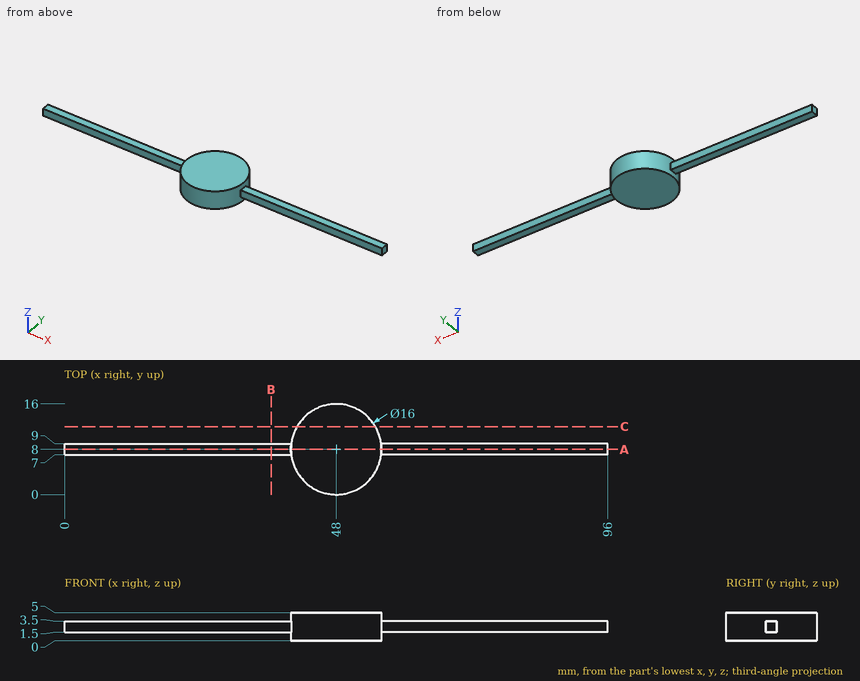
Input: dimensioned drawing with shaded views. Units: mm. Origin: part minimum x, y, z. Coordinates: 2 decimals unless noted, no trailing zeros. Loops run counter-clockwise (first coordinate to the right, second up) from the corner with the lowest first, then second, coordinate; pieces in that order, holes last. Notation, with made-up numbers: M 10.5,37.5 L 69.5,37.5 A29 ccw 69.5,67.5 Z; hole C -24,-25.5 d3. An arc over 180 degrees is marked long. One line per item, written item: value. Start each with the question number.
1) Material intervals for L1, parallel to Y at x = 5, z = 1.55; L2, parallel to X at y = 8, z = 4.15; L3, parallel to X at y = 13.25, z = 1.85, sorted ascending. Write a range as from..to.
2) Pin query (flat end, axial travel): P1, Ø2, axis at x = 77.5, z = 2.5, coming from the +Y side; P2, Ø0.6, axis at x = 14, y = 7.5, coming from the -Z side; P3, Ø2, axis at x = 17.5, z = 2.5, coming from the -Y side. Return the tip coordinate at first contact, or that it passes through.
3) Cut plane A-A (y = 8). Return loops of the section in (x, z).
4) Cut plane C-C (y = 12). Return loops of the section in (x, z).
5) Cut plane B-B (x = 36.5). Return loops of the section in (y, z).
Evaluation:
1. L1: 7..9
1. L2: 40..56
1. L3: 41.96..54.04
2. P1: y = 9
2. P2: z = 1.5
2. P3: y = 7
3. outline: M 0,1.5 L 40,1.5 L 40,0 L 56,0 L 56,1.5 L 96,1.5 L 96,3.5 L 56,3.5 L 56,5 L 40,5 L 40,3.5 L 0,3.5 Z
4. outline: M 41.07,0 L 54.93,0 L 54.93,5 L 41.07,5 Z
5. outline: M 7,1.5 L 9,1.5 L 9,3.5 L 7,3.5 Z
